Input: part model. Units: mm. Frame: model coordinates. Face numbers are marked on the shaded views. A direction names the side the tool comes from. Coordinates: 2 decimals unless noted, no trailing zeros. Write each loop counter-clockwise with the first axis right and the second up, starting at its lowest first coordinate (ties: lowest second). Pieces come first, ordered by that corner, then holes. Notation, with made-up numbers: M 75.5,31.25 L 79.5,31.25 A15 cw 79.5,35.25 Z; hole C 54,43 d11. An arc over 180 degrees is marked long. Use CSV: the item, a comma, the result in double quotes.
```python
from build123d import *

# Parameters (mm, degrees)
F4_DEPTH = 3
F7_DEPTH = 2.5


with BuildPart() as f1:
    # F0 (on Front) → F1 (revolve)
    with BuildSketch(Plane.XZ):
        Polygon((2.250003, 6), (2.250003, 0), (64.250003, 0), (81.750003, 0), (81.750003, 6), (64.250003, 6), (60.850003, 6), (60.850003, 5.75), (59.750003, 5.75), (59.750003, 6), (51.750003, 6), (51.750003, 8.5), (49.350003, 8.5), (49.350003, 8.1), (48.250003, 8.1), (48.250003, 8.5), (18.250003, 8.5), (18.250003, 8.1), (17.150003, 8.1), (17.150003, 8.5), (14.750003, 8.5), (14.750003, 6), (6.750003, 6), (6.750003, 5.75), (5.650003, 5.75), (5.650003, 6), align=None)
    revolve(axis=Axis((33.250003, 0, 0), (1, 0, 0)))

    # F3 (on offset) → F4 (cut)
    with BuildSketch(Plane.XY.offset(8.5)):
        with BuildLine():
            Line((43.250003, 2.5), (23.250003, 2.5))
            ThreePointArc((23.250003, 2.5), (20.750003, 0), (23.250003, -2.5))
            Line((23.250003, -2.5), (43.250003, -2.5))
            ThreePointArc((43.250003, -2.5), (45.750003, 0), (43.250003, 2.5))
        make_face()
    extrude(amount=-F4_DEPTH, mode=Mode.SUBTRACT)

    # F6 (on offset) → F7 (cut)
    with BuildSketch(Plane.XY.offset(6)):
        with BuildLine():
            Line((82.259692, 2), (63.750003, 2))
            ThreePointArc((63.750003, 2), (61.750003, 0), (63.750003, -2))
            Line((63.750003, -2), (82.259692, -2))
            Line((82.259692, -2), (82.259692, 2))
        make_face()
    extrude(amount=-F7_DEPTH, mode=Mode.SUBTRACT)


solid = f1.part
```
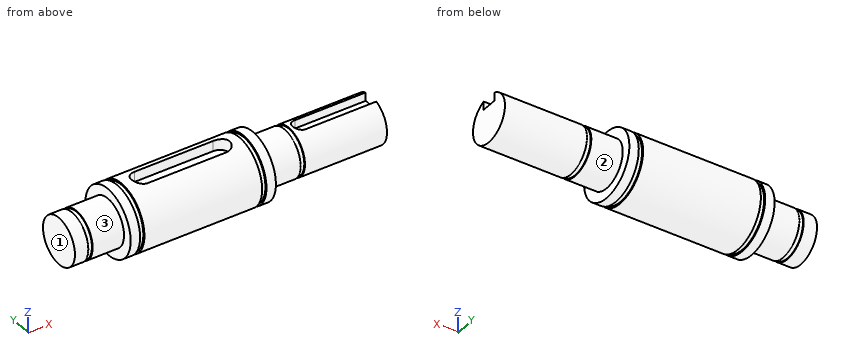
1. Contact query for flat-ended pins moving along their axis: pin 1 Ø6 at (x, y) = (10.5, 3) entering from +Z; pin 2 Ø4 at (x, z) = (11.5, -7) entering from -Y; pin 3 Ø10 at (x, z) = (70.5, -5.5) entering from -Y; pin 4 Ø8.5 at (y, z) = (-1.5, 4) entering from +X. Output: stop coordinate, or through.
Resolved:
pin 1,"stops at z = 6"
pin 2,"stops at y = -3.32"
pin 3,"stops at y = -5.98"
pin 4,"stops at x = 81.75"
2. Access query for the marked faces 1, 2 and 3. Directions: +Z, -Z, +X, -X, +Y, -Y. A direction counts if a zero-diameter tool reaches every point of the face in a straight line with its end or side. Return the directions, or none.
Resolved:
face 1,"+Z, -Z, -X, +Y, -Y"
face 2,"+X"
face 3,"-X"
3. Section B-B (x = 44.5). Return loops of the section in (y, z), then the cut area to 3 significant figures.
Resolved:
outline,"M -2.17,5.5 L -2.17,8.22 A8.5 ccw long 2.17,8.22 L 2.17,5.5 Z"
area,"214 mm^2"
4. Section C-C (x = 67). Return loops of the section in (y, z), then the cut area to 3 significant figures.
Resolved:
outline,"M -2,3.5 L -2,5.66 A6 ccw long 2,5.66 L 2,3.5 Z"
area,"104 mm^2"
5. Material intervals for line 1 (X direction, y = 3.25, z = -5); line 2 (Y direction, x = 28, z = -6.25); line 3 (Y direction, x = 62.5, z = 5.5), sorted ascending. Write a range as [from, to].
Resolved:
line 1,"x = [2.25, 5.65], [6.75, 59.75], [60.85, 81.75]"
line 2,"y = [-5.76, 5.76]"
line 3,"y = [-2.4, -1.56], [1.56, 2.4]"
6. Section A-A (x = 58). Return loops of the section in (y, z), then the cut area to 3 significant figures.
Resolved:
outline,"C 0,0 d12"
area,"113 mm^2"
